Could you check a few things on this model? Use its own coordinates, in mm. A direction names the side the tool comes from. Coordinates: 2 decimals unless noted, no trailing zeros. Write each loop counter-clockwise with the first axis right and the second up, starting at its lowest first coordinate (ties: lowest second). Pieces come first, ordered by that corner, then holes. Notation, with made-up numbers: (-40, -5) - (0, -5) arc R17 cw to (0, 17) - close; hole circle Ø11 at (19, 44.5). An arc over 180 degrees is marked (long way). Answer as a JSON object with one key per item and string values. Group by question number.
1) Please list where these lines run through material, in increasing order: line 1 along Z through (x, y) = (32, 29); line 2 along Z through (x, y) = (-17, -50); line 3 along Y through (x, z) = (2, -1.5).
2) We'd pull the mould along X, two halves only. Please class faces 5 (the cylindrical face through (-53, 0, 34)), 6 (the flat face through (9, -19, 39.5)), 7 (the flat face through (5, 0, 59)): released by +X, released by -X, zero draft, split by the parting line, or undercut.
3) Will these pins go through, and if not, where does the flat tip stop? pin 1 Ø7.5 at (y, z) = (-0.5, 60) entering from +X; pin 2 Ø8 at (x, y) = (-45.5, 3) entering from -Z; pin 3 Ø0.5 at (x, y) = (5.5, 1) entering from +Z.
4) If we section it at B-B (z = -54): Write out the boundary of the cut face in (x, y).
5) If we section it at A-A (z = 13): Write out the boundary of the cut face in (x, y).
6) On a 3-axis mill with a long thin cutter (end or side, diameter ignored), from which of +Z, -Z, +X, -X, +Y, -Y can I reach the whole of each face in a straight line? I mean faces 1 (the cylindrical face through (20.765, 39.923, 33.416)), 2 (the flat face through (-50, 0, 39.5)), 3 (the flat face through (-1.1, 6.1, -48)), 4 (the flat face through (-25, -43, 39.5)). Say none if no direction works.
Autodesk Inventor part; units mm, degrees
ref_plane "YZ Plane" through (0, 0, 0) normal (1, 0, 0) x (0, 1, 0)
ref_plane "XZ Plane" through (0, 0, 0) normal (0, 1, 0) x (-1, 0, 0)
ref_plane "XY Plane" through (0, 0, 0) normal (0, 0, 1) x (1, 0, 0)
sketch "スケッチ1" plane through (0, 0, 0) normal (0, 0, 1) x (1, 0, 0)
  circle A0 centre (0, 0) radius 6
  dimension "d0" = 12
extrude "押し出し1" add sketch "スケッチ1" along normal mid plane 132
sketch "スケッチ2" plane through (0, 0, 0) normal (0, 0, 1) x (1, 0, 0)
  circle A0 centre (0, 0) radius 6 construction
  circle A1 centre (0, 0) radius 7.4
  dimension "d3" = 14.8
extrude "押し出し2" add sketch "スケッチ2" along normal mid plane 96
sketch "スケッチ3" plane through (0, 0, 0) normal (0, 0, 1) x (1, 0, 0)
  circle A0 centre (0, 0) radius 6
  circle A1 centre (0, 0) radius 19.65
  dimension "d6" = 39.3
extrude "押し出し3" add sketch "スケッチ3" along normal mid plane 92
sketch "スケッチ4" plane through (0, 0, 0) normal (0, 0, 1) x (1, 0, 0)
  circle A0 centre (0, 0) radius 45
  dimension "d9" = 90
extrude "押し出し4" add sketch "スケッチ4" along normal mid plane 79
sketch "スケッチ5" plane through (0, 0, 0) normal (0, 0, 1) x (1, 0, 0)
  circle A0 centre (0, 0) radius 58.5
  dimension "d12" = 117
extrude "押し出し5" add sketch "スケッチ5" along normal mid plane 55
fillet "フィレット1" radius 5 2 edges at (-58.5, 0, 27.5) (-58.5, 0, -27.5)
sketch "スケッチ6" plane through (0, 0, 39.5) normal (0, 0, 1) x (1, 0, 0)
  circle A0 centre (0, 0) radius 50 construction
  circle A1 centre (50, 0) radius 3
  circle A2 centre (25, 43.3013) radius 3
  circle A3 centre (-25, 43.3013) radius 3
  circle A4 centre (-50, 0) radius 3
  circle A5 centre (-25, -43.3013) radius 3
  circle A6 centre (25, -43.3013) radius 3
  dimension "d16" = 100
  dimension "d17" = 6
  dimension "d20" = 360
extrude "押し出し6" add sketch "スケッチ6" against normal up to surface (12 mm away)
sketch "スケッチ7" plane through (0, 0, 66) normal (0, 0, 1) x (1, 0, 0)
  circle A0 centre (0, 0) radius 6
  line L0 (-5, 3.3166) -> (-5, -3.3166)
  circle A1 centre (0, 0) radius 6
  line L1 (5, 3.3166) -> (5, -3.3166)
  dimension "d24" = 5
  dimension "d25" = 5
extrude "押し出し7" cut sketch "スケッチ7" against normal blind 15 contours A0 L1 | L0 A0
properties part number "movero"
Here are the results:
{
 "1": {"line 1": "z = -39.5 to 39.5", "line 2": "z = -27.5 to 27.5", "line 3": "y = -58.47 to 58.47"},
 "2": {"face 5": "undercut", "face 6": "zero draft", "face 7": "released by +X"},
 "3": {"pin 1": "stops at x = 5", "pin 2": "stops at z = -39.5", "pin 3": "stops at z = 51"},
 "4": {"outline": "circle Ø12 at (0, 0)"},
 "5": {"outline": "circle Ø117 at (0, 0)"},
 "6": {"face 1": "+Z", "face 2": "+Z, -X, +Y, -Y", "face 3": "-Z", "face 4": "+Z, +X, -X, +Y, -Y"}
}
